Autodesk Inventor part; units mm, degrees
ref_plane "YZ Plane" through (0, 0, 0) normal (1, 0, 0) x (0, 1, 0)
ref_plane "XZ Plane" through (0, 0, 0) normal (0, 1, 0) x (-1, 0, 0)
ref_plane "XY Plane" through (0, 0, 0) normal (0, 0, 1) x (1, 0, 0)
sketch "Boceto1" plane through (0, 0, 0) normal (0, 1, 0) x (-1, 0, 0)
  line L0 (0, 35) -> (0, -35) construction
  line L1 (25, 35) -> (25, -35)
  line L2 (-25, -35) -> (-25, 35)
  arc A0 (25, 35) -> (-25, 35) centre (0, 35) ccw
  arc A1 (-25, -35) -> (25, -35) centre (0, -35) ccw
  circle A2 centre (0, -35) radius 15
  circle A3 centre (0, 35) radius 15
  line L3 (0, -20) -> (0, -20)
  line L4 (15, -35) -> (-15, -35)
  line L5 (94.5074, 0) -> (-76.0102, 0) construction
  line L6 (15, 35) -> (-15, 35)
  line L7 (15, -35) -> (-15, -35)
  circle A4 centre (0, 10) radius 15
  circle A5 centre (0, -10) radius 15
  point P0 (0, 0)
  point P1 (0, 60)
  point P2 (0, -60)
  point P3 (0, -20)
  point P4 (15, 35)
  point P5 (11.1803, 0)
  point P6 (-11.1803, 0)
  dimension "largo" = 120
  dimension "ancho" = 50
  dimension "espesor_junta" = 10
  dimension "d3" = 10
  dimension "d6" = 0
  dimension "d22" = 30
  dimension "d23" = 30
  dimension "d24" = 20
  dimension "d25" = 10
extrude "Extrusión6" add sketch "Boceto1" along normal blind 10 contours L1 A1 L2 A0 | A2 A5 L4 | A3 L6 A4
equation "\"d3\" = espesor_junta"
properties part number "mod4" material "Aluminio 6061"
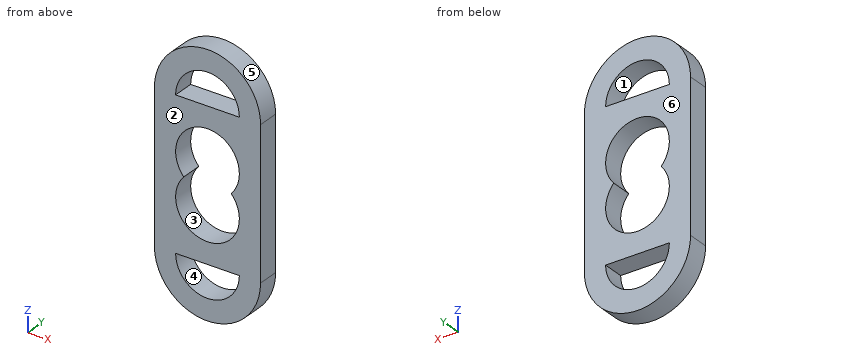
Verification items for the finished model (mm, model axes). Face numbers are marked on the shaded views. A direction names the side the tool comes from. Coordinates: 2 decimals unless noted, no trailing zeros. Write each loop counter-clockwise with the first axis right and the second up, starting at its lowest first coordinate (ties: lowest second). Pieces come first, ordered by that corner, then holes. Notation, with made-up numbers: (-5.75, 19) - (0.25, 19) arc R33 ccw to (0.25, 58) - close; hole circle Ø6 at (-33, 42). An arc over 180 degrees is marked (long way). Answer as a JSON object with one key per item and string values.
(1) Cross-section at C-C on y = 6.5. Record the cut outline in (x, z), plus the area to 3 significant figures.
Report:
{"outline": "(-25, -35) arc R25 ccw to (25, -35) - (25, 35) arc R25 ccw to (-25, 35) - close; hole (-15, -35) arc R15 ccw to (15, -35) - close; hole (-15, 35) - (15, 35) arc R15 ccw to start; hole (-11.18, 0) arc R15 ccw (long way) to (11.18, 0) arc R15 ccw (long way) to start", "area": "3,500 mm^2"}
(2) Cross-section at B-B on z = -10. Record the cut outline in (x, y).
Report:
{"outline": "(-25, 0) - (-15, 0) - (-15, 10) - (-25, 10) - close; (15, 0) - (25, 0) - (25, 10) - (15, 10) - close"}
(3) Gauge pin test, flat end, axial feed: pin 1 Ø1.5 at (x, y) = (2, 9) entering from -Z. Record the tip position at first contact, or that the pin passes through.
Report:
{"pin 1": "z = -59.97"}
(4) Cross-section at A-A on x = 0. Record the cut outline in (y, z), plus the area to 3 significant figures.
Report:
{"outline": "(0, -60) - (10, -60) - (10, -50) - (0, -50) - close; (0, -35) - (10, -35) - (10, -25) - (0, -25) - close; (0, 25) - (10, 25) - (10, 35) - (0, 35) - close; (0, 50) - (10, 50) - (10, 60) - (0, 60) - close", "area": "400 mm^2"}
(5) Mould release check, pull along X, two halves, no side actions. Record for the marked faces 3, 4, 5 and 6: pulls with the +X half, pulls with the -X half, needs draft (parallel to the pull), parting line crosses it, or undercut.
Report:
{"face 3": "undercut", "face 4": "undercut", "face 5": "parting line crosses it", "face 6": "needs draft"}
(6) Thickness scan on line 1 along Z through (x, y) = (0, 5.75); line 2 along X through (y, z) = (4, 10); line 3 along Z through (x, y) = (-13, 7.75). Record the ranges inside material, lowest first.
Report:
{"line 1": "-60 to -50, -35 to -25, 25 to 35, 50 to 60", "line 2": "-25 to -15, 15 to 25", "line 3": "-56.35 to -42.48, -35 to -17.48, -2.52 to 2.52, 17.48 to 35, 42.48 to 56.35"}
(7) Tool access check on the marked faces 1 and 2. Record the directions out of +Z, -Z, +X, -X, +Y, -Y that give a thin tool (end or side, any length) a straight path to the whole face; none if there is none.
Report:
{"face 1": "+Y, -Y", "face 2": "+Z, -Z, +X, -X, -Y"}
(8) Cross-section at D-D on z = 11. Record the cut outline in (x, y), plus the area to 3 significant figures.
Report:
{"outline": "(-25, 0) - (-14.97, 0) - (-14.97, 10) - (-25, 10) - close; (14.97, 0) - (25, 0) - (25, 10) - (14.97, 10) - close", "area": "201 mm^2"}
